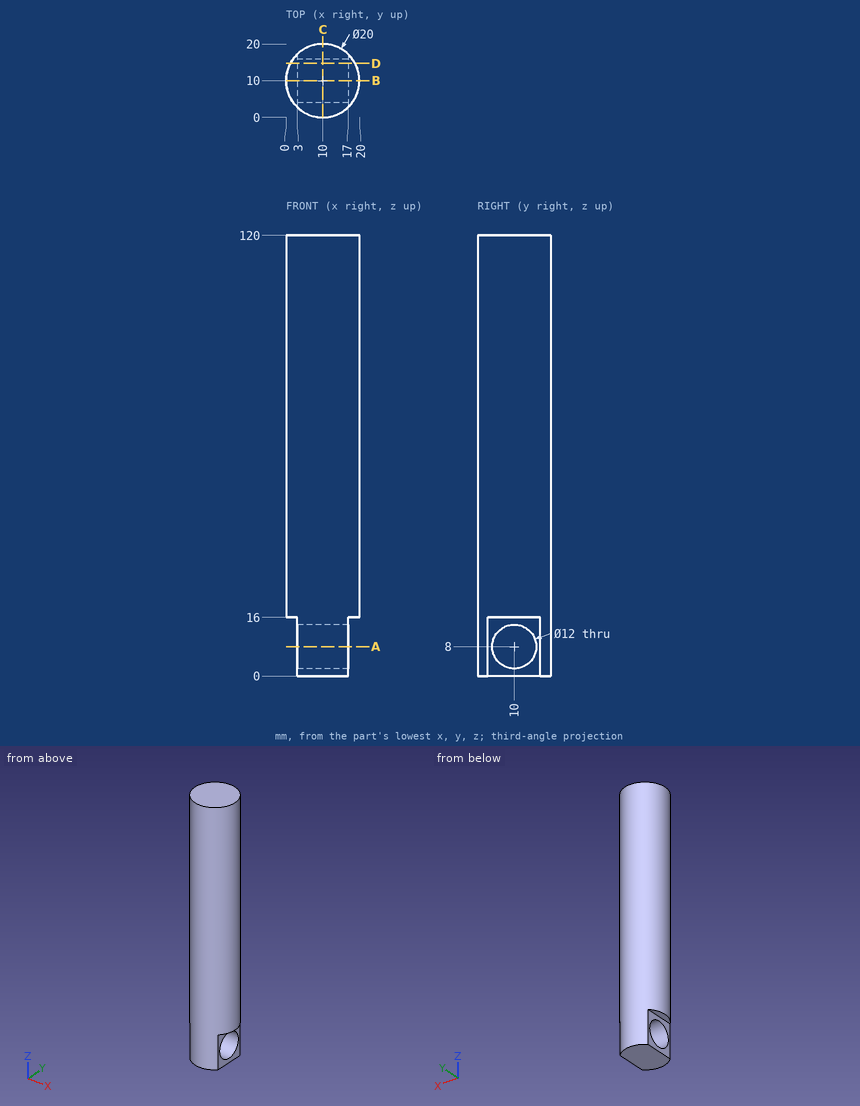
The figure shows three views and two pictorial views of one solid part (mm, origin at its lowest corner). Answer the questions. Give positions to 0.01 mm unless a question says otherwise; leave off trailing zeros. Write each loop counter-clockwise with the first axis right and the second up, starting at its lowest first coordinate (ties: lowest second). Pieces come first, ordered by that corner, then holes. Notation, with made-up numbers: (36, 34.5) -> (68, 34.5) arc R23 ccw to (68, 63.5) -> close; hole circle Ø4 at (-27, 81). An arc over 180 degrees is marked (long way). Use one line per item in the form item = value.
1) Each of these flat-tipped pins is pushed along its axis until it touches: P1, Ø6, axis at x = 5.5, z = 13, coming from the +Y side; P2, Ø6, axis at x = 17, z = 32.5, coming from the -Y side; P3, Ø2.5, axis at x = 1.5, y = 9.5, coming from the -Z side; P4, Ø4.5, axis at y = 10.5, z = 9.5, coming from the +X side. Where does it stop, or does it pass through?
Result:
P1 = 19.89
P2 = 0.83
P3 = 16
P4 = through
2) Straight lines are drawn through the part: probe 1 along Y at (x, z) = (10.5, 8); probe 2 along Z at (x, y) = (13.5, 10); probe 3 along Z at (x, y) = (13.75, 8.5). For each, find the intervals that lie inside material, in ascending order.
Result:
probe_1 = 0.01 to 4, 16 to 19.99
probe_2 = 0 to 2, 14 to 120
probe_3 = 0 to 2.19, 13.81 to 120
3) Section C-C on x = 10 is taken. Write down the section's boundary in (y, z).
Result:
outline = (0, 0) -> (20, 0) -> (20, 120) -> (0, 120) -> close; hole circle Ø12 at (10, 8)
4) Section B-B on y = 10 is taken. Write down the section's boundary in (x, z).
Result:
outline = (0, 16) -> (3, 16) -> (3, 14) -> (17, 14) -> (17, 16) -> (20, 16) -> (20, 120) -> (0, 120) -> close; (3, 0) -> (17, 0) -> (17, 2) -> (3, 2) -> close
5) Section D-D on y = 14.75 is taken. Write down the section's boundary in (x, z), plus the area to 3 significant figures.
Result:
outline = (1.2, 16) -> (3, 16) -> (3, 11.67) -> (17, 11.67) -> (17, 16) -> (18.8, 16) -> (18.8, 120) -> (1.2, 120) -> close; (3, 0) -> (17, 0) -> (17, 4.33) -> (3, 4.33) -> close
area = 1,950 mm²
6) Section A-A on z = 8 is taken. Write down the section's boundary in (x, y), plus the area to 3 significant figures.
Result:
outline = (3, 2.86) arc R10 ccw to (17, 2.86) -> (17, 4) -> (3, 4) -> close; (3, 16) -> (17, 16) -> (17, 17.14) arc R10 ccw to (3, 17.14) -> close
area = 87.1 mm²
